Read the model definition and answer for the solid it produces. Units are mm, in the model's axes. Round coordinates to 2 decimals unless told otherwise and drop trailing zeros. Order: outer loops, then holes, each group sorted by start corner. A loop starts at its lowest first (then second) coordinate and runs counter-clockwise, first axis right, second up. Notation, with made-up numbers: (-28, 52) -> (25, 52) arc R9 ccw to (25, 62) -> close; hole circle Ø7 at (-7, -1.5). An arc over 180 degrees is marked (long way). Use a Markdown table: item, result. Add a question column.
1. Section A-A, the plane x = -20 is taken. Give the vertices of the cut face in (y, z).
2. Given pin 1 (1.5 mm diameter, centred on x = -37, z = 2.5, fed in from -Y); pin 2 (1.5 mm diameter, centred on y = -20, z = 3, fed in from -X); pin 3 (1.5 mm diameter, centred on y = -44, z = 0.5, fed in from -X), each flat-ended and moving along its own axis, determine where each tip first touches the part or whether it passes through.
3. Section C-C, the plane x = -49 is taken. Give the vertices of the cut face in (y, z).
4. Consider L1, parallel to X at y = -68, z = 3.45; L2, parallel to Y at x = -101.5, z = 0.55; L3, parallel to Y at x = -35.5, z = 1.9. Determine where each line is inside the solid, lowest interval first. Write a range as [from, to].
5. Section B-B, the plane y = -20 is taken. Give the vertices of the cut face in (x, z), then the cut area to 3 significant figures.
6. Section D-D, the plane y = -119 is taken. Give the vertices of the cut face in (x, z), then the cut area to 3 significant figures.
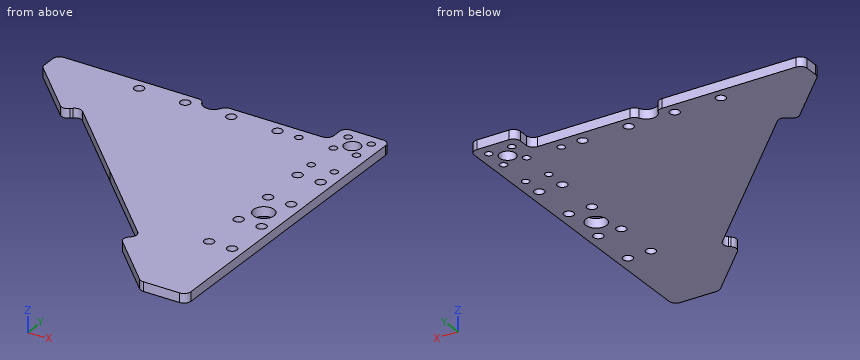
```python
from build123d import *

# Parameters (mm, degrees)
SKETCH_1_W          = 118
SKETCH_1_H          = 20
SKETCH_1_W_2        = 20
SKETCH_1_H_2        = 118
EXTRUDE_1_DEPTH     = 4
SKETCH_3_R          = 3.5
SKETCH_3_R_2        = 1.6
CUT_EXTRUDE_1_DEPTH = 4
SKETCH_4_R          = 4.5
SKETCH_4_R_2        = 2.1
CUT_EXTRUDE_2_DEPTH = 4
CUT_EXTRUDE_7_DEPTH = 4
SKETCH_12_W         = 118
SKETCH_12_H         = 10
CUT_EXTRUDE_8_DEPTH = 4
FILLET_3_R          = 3


with BuildPart() as part:
    # 草图1 → 凸台-拉伸1 (new body)
    with BuildSketch(Plane.XY):
        with Locations((-69, 0)):
            Rectangle(SKETCH_1_W, SKETCH_1_H)
        Rectangle(SKETCH_1_W_2, SKETCH_1_H)
        with Locations((0, -69)):
            Rectangle(SKETCH_1_W_2, SKETCH_1_H_2)
        Polygon((-128, -10), (-10, -10), (-10, -128), align=None)
    extrude(amount=EXTRUDE_1_DEPTH)

    # 草图3 → 切除-拉伸1 (cut)
    with BuildSketch(Plane.XY.offset(4)):
        Circle(SKETCH_3_R)
        with Locations((5, 5)):
            Circle(SKETCH_3_R_2)
        with Locations((-5, 5)):
            Circle(SKETCH_3_R_2)
        with Locations((-5, -5)):
            Circle(SKETCH_3_R_2)
        with Locations((5, -5)):
            Circle(SKETCH_3_R_2)
        with Locations((-20, -5)):
            Circle(SKETCH_3_R_2)
        with Locations((-5, -20)):
            Circle(SKETCH_3_R_2)
        with Locations((5, -20)):
            Circle(SKETCH_3_R_2)
        with Locations((5, 20)):
            Circle(SKETCH_3_R_2)
        with Locations((-5, 20)):
            Circle(SKETCH_3_R_2)
        with Locations((20, -5)):
            Circle(SKETCH_3_R_2)
        with Locations((20, 5)):
            Circle(SKETCH_3_R_2)
        with Locations((-20, 5)):
            Circle(SKETCH_3_R_2)
    extrude(amount=-CUT_EXTRUDE_1_DEPTH, mode=Mode.SUBTRACT)

    # 草图4 → 切除-拉伸2 (cut)
    with BuildSketch(Plane.XY.offset(4)):
        with Locations((0, -60)):
            Circle(SKETCH_4_R)
        with Locations((-5, -29.263884189)):
            Circle(SKETCH_4_R_2)
        with Locations((5, -29.263884189)):
            Circle(SKETCH_4_R_2)
        with Locations((5, -49.263884189)):
            Circle(SKETCH_4_R_2)
        with Locations((5, -69.263884189)):
            Circle(SKETCH_4_R_2)
        with Locations((5, -89.263884189)):
            Circle(SKETCH_4_R_2)
        with Locations((-5, -49.263884189)):
            Circle(SKETCH_4_R_2)
        with Locations((-5, -69.263884189)):
            Circle(SKETCH_4_R_2)
        with Locations((-5, -89.263884189)):
            Circle(SKETCH_4_R_2)
        with Locations(Location((-89.263884189, -5, 0), (0, 0, 180))):
            Circle(SKETCH_4_R_2)
        with Locations(Location((-69.263884189, -5, 0), (0, 0, 180))):
            Circle(SKETCH_4_R_2)
        with Locations(Location((-49.263884189, -5, 0), (0, 0, 180))):
            Circle(SKETCH_4_R_2)
        with Locations(Location((-89.263884189, 5, 0), (0, 0, 180))):
            Circle(SKETCH_4_R_2)
        with Locations(Location((-69.263884189, 5, 0), (0, 0, 180))):
            Circle(SKETCH_4_R_2)
        with Locations(Location((-49.263884189, 5, 0), (0, 0, 180))):
            Circle(SKETCH_4_R_2)
        with Locations(Location((-29.263884189, 5, 0), (0, 0, 180))):
            Circle(SKETCH_4_R_2)
        with Locations(Location((-29.263884189, -5, 0), (0, 0, 180))):
            Circle(SKETCH_4_R_2)
        with Locations(Location((-60, 0, 0), (0, 0, 180))):
            Circle(SKETCH_4_R)
    extrude(amount=-CUT_EXTRUDE_2_DEPTH, mode=Mode.SUBTRACT)

    # 草图11 → 切除-拉伸7 (cut)
    with BuildSketch(Plane.XY.offset(4)):
        Polygon((-69, -69), (-64.050252532, -64.050252532), (-99.405591591, -28.694913472), (-104.355339059, -33.644660941), align=None)
        Polygon((-28.694913472, -99.405591591), (-64.050252532, -64.050252532), (-69, -69), (-33.644660941, -104.355339059), align=None)
    extrude(amount=-CUT_EXTRUDE_7_DEPTH, mode=Mode.SUBTRACT)

    # 草图12 → 切除-拉伸8 (cut)
    with BuildSketch(Plane.XY.offset(4)):
        with Locations((-69, 5)):
            Rectangle(SKETCH_12_W, SKETCH_12_H)
    extrude(amount=-CUT_EXTRUDE_8_DEPTH, mode=Mode.SUBTRACT)

    # 圆角3
    fillet_3_edges = [part.edges().sort_by_distance(p)[0] for p in [
        (10, 10, 2),
        (10, -128, 2),
        (-10, -128, 2),
        (-128, -10, 2),
        (-99.405591591, -28.694913472, 2),
        (-28.694913472, -99.405591591, 2),
        (-33.644660941, -104.355339059, 2),
        (-104.355339059, -33.644660941, 2),
        (-64.5, 0, 2),
        (-55.5, 0, 2),
        (-10, 0, 2),
        (-128, 0, 2),
        (-10, 10, 2),
    ]]
    fillet(fillet_3_edges, radius=FILLET_3_R)


solid = part.part
```
Verdict:
| question | item | result |
|---|---|---|
| 1 | outline | (-118, 0) -> (-6.6, 0) -> (-6.6, 4) -> (-118, 4) -> close; (-3.4, 0) -> (0, 0) -> (0, 4) -> (-3.4, 4) -> close |
| 2 | pin 1 | stops at y = -91.85 |
| 2 | pin 2 | stops at x = -118.75 |
| 2 | pin 3 | stops at x = -84.85 |
| 3 | outline | (-79.1, 0) -> (-7.08, 0) -> (-7.08, 4) -> (-79.1, 4) -> close; (-2.92, 0) -> (0, 0) -> (0, 4) -> (-2.92, 4) -> close |
| 4 | L1 | x = [-60.1, -6.68], [-3.32, 3.32], [6.68, 10] |
| 4 | L2 | y = [-30.79, 0] |
| 4 | L3 | y = [-92.6, 0] |
| 5 | outline | (-118, 0) -> (-6.6, 0) -> (-6.6, 4) -> (-118, 4) -> close; (-3.4, 0) -> (3.4, 0) -> (3.4, 4) -> (-3.4, 4) -> close; (6.6, 0) -> (10, 0) -> (10, 4) -> (6.6, 4) -> close |
| 5 | area | 486 mm2 |
| 6 | outline | (-19, 0) -> (10, 0) -> (10, 4) -> (-19, 4) -> close |
| 6 | area | 116 mm2 |
